Design review of the part shown in the three views and the two pictorial views. Dimensions are in mm from the part's minimum x, y and z. A direction names the side the tool comes from. Coordinates: 2 decimals unless noted, no trailing zeros. Loops run counter-clockwise (first coordinate to the right, second up) from the corner with the lowest first, then second, coordinate; pieces in that order, holes last. Notation, with made-up numbers: (43, 14.25) -> (76, 14.25) arc R26 cw to (76, 41.25) -> close; hole circle Ø11 at (62, 9.5). An arc over 180 degrees is marked (long way). Answer in a Markdown table with one row per item.
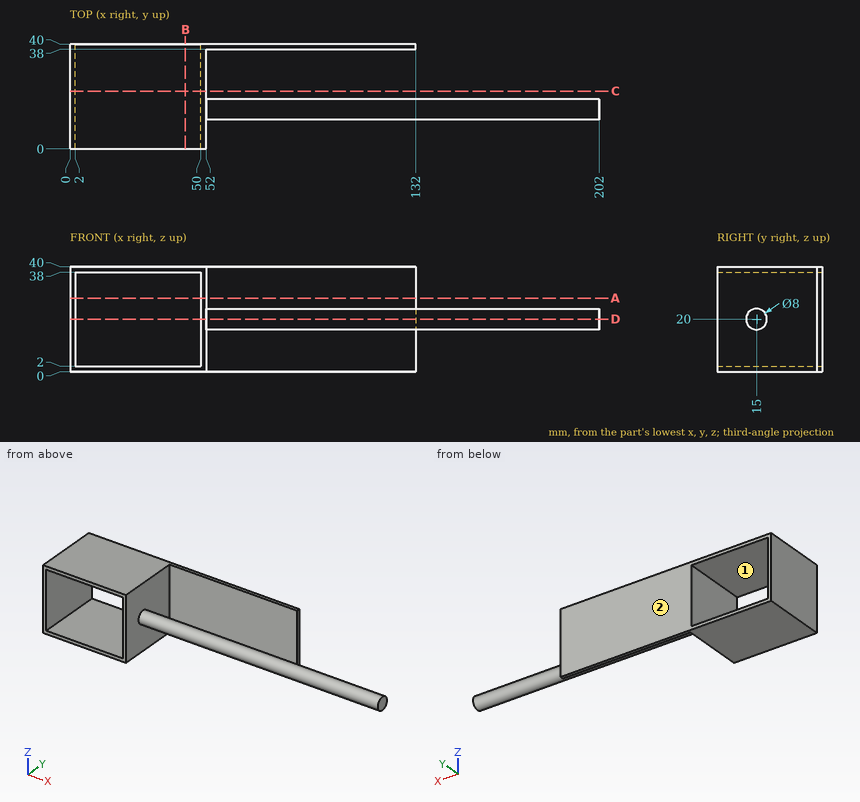
Item 1: Insertion check: pin 1 (12 mm diameter, centred on x = 25, z = 34.5, fed in from -Y); pin 2 (5 mm diameter, centred on x = 178, y = 17, fed in from -Z); pin 3 (8 mm diameter, centred on x = 159.5, y = 15.5, fed in from +Z); pin 4 (8 mm diameter, centred on y = 30.5, z = 14, fed in from +X). Each pin has a flat end and moves straight along its axis. Give the tip position at first contact, or say it passes through.
Worked answers:
| item | result |
|---|---|
| pin 1 | y = 0 |
| pin 2 | z = 16 |
| pin 3 | z = 24 |
| pin 4 | x = 52 |
Item 2: For the marked faces 1 and 2, list the 3-axis set-ups (+Z, -Z, +X, -X, +Y, -Y) from which the entire face can be reached by the end or side of a thin tool; tool diameter is ignored.
Worked answers:
| item | result |
|---|---|
| face 1 | +Y, -Y |
| face 2 | +Z, -Z, +X, -X, +Y |
Item 3: For L1, parallel to Z at x = 31.5, y = 30.5; L2, parallel to X at y = 4.5, z = 22.5; L3, parallel to Y at x = 87, z = 36, list the stretches that pass through material, from the lowest coordinate up.
Worked answers:
| item | result |
|---|---|
| L1 | 0 to 2, 38 to 40 |
| L2 | 0 to 2, 50 to 52 |
| L3 | 38 to 40 |
Item 4: Take a section at C-C, the plane y = 22. State the section outline as (x, z) points, and give its area (3 significant figures).
Worked answers:
| item | result |
|---|---|
| outline | (0, 0) -> (52, 0) -> (52, 40) -> (0, 40) -> close; hole (2, 2) -> (50, 2) -> (50, 38) -> (2, 38) -> close |
| area | 352 mm² |
Item 5: Take a section at B-B, the plane x = 44. State the section outline as (y, z) points, and give its area (3 significant figures).
Worked answers:
| item | result |
|---|---|
| outline | (0, 0) -> (40, 0) -> (40, 2) -> (0, 2) -> close; (0, 38) -> (40, 38) -> (40, 40) -> (0, 40) -> close |
| area | 160 mm² |
Item 6: Take a section at A-A, the plane z = 28. State the section outline as (x, y) points, and give its area (3 significant figures).
Worked answers:
| item | result |
|---|---|
| outline | (0, 0) -> (2, 0) -> (2, 40) -> (0, 40) -> close; (50, 0) -> (52, 0) -> (52, 38) -> (132, 38) -> (132, 40) -> (50, 40) -> close |
| area | 320 mm² |
Item 7: Take a section at D-D, the plane z = 20. State the section outline as (x, y) points, and give its area (3 significant figures).
Worked answers:
| item | result |
|---|---|
| outline | (0, 0) -> (2, 0) -> (2, 40) -> (0, 40) -> close; (50, 0) -> (52, 0) -> (52, 11) -> (202, 11) -> (202, 19) -> (52, 19) -> (52, 38) -> (132, 38) -> (132, 40) -> (50, 40) -> close |
| area | 1,520 mm² |
